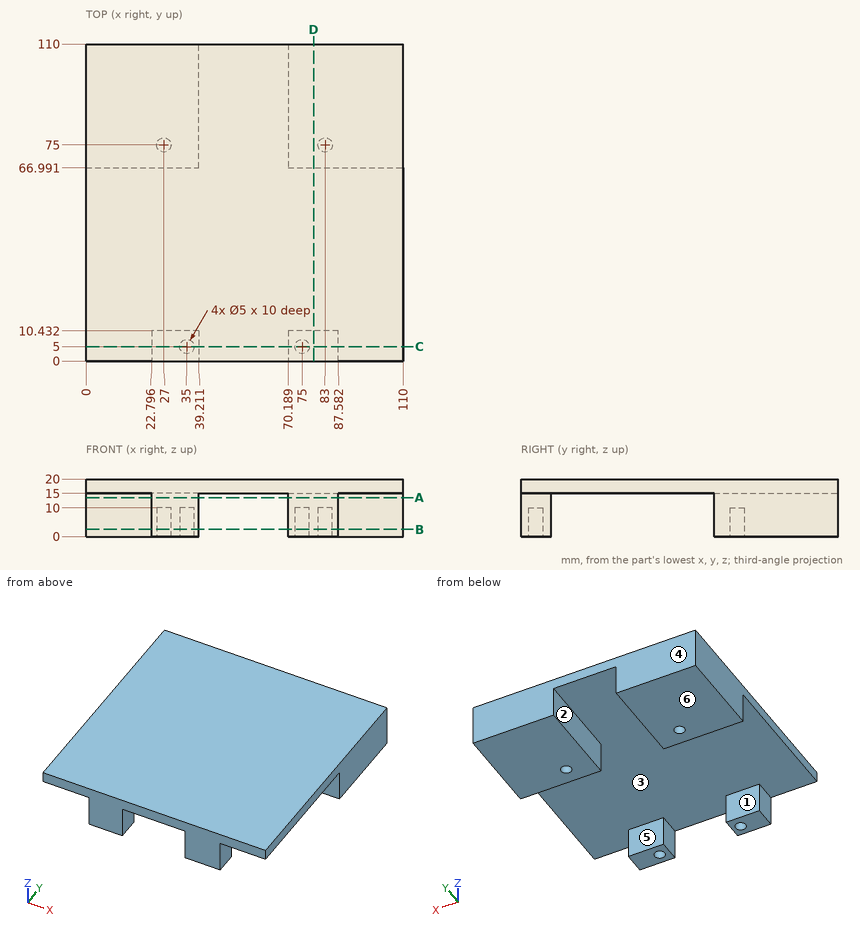
Here's the drawing with two shaded views (mm, measured from the low corner). I have some questions. A direction names the side the tool comes from. Give positions to 0.01 mm unless a question says otherwise; leave off trailing zeros. Write each loop counter-clockwise with the first axis right and the second up, starting at its lowest first coordinate (ties: lowest second). Pieces come first, ordered by that corner, then holes. Notation, with made-up numbers: (33, 14.25) -> (49, 14.25) arc R35 ccw to (49, 51.25) -> close; hole circle Ø10 at (-4, 57.25). An arc over 180 degrees is marked (long way). Answer as a JSON object with one key per item and string values. Group by question number.
Item 1: We'd pull the mould along Y, two halves only. Please class the marked faces 4, 5 and 6: +Y half, -Y half, draft (parallel to the pull), parting line (faces both ways), or undercut.
Item 2: Suppose I cut it at D-D (x = 79). Please give me the cut outline in (y, z), plus the area to 3 significant figures.
Item 3: Please list where these lines run through material, in increasing order: line 1 (X direction, y = 75, z = 3.5); line 2 (X direction, y = 5, z = 2) (1 decimal); line 3 (X direction, y = 72, z = 12.75). Write a range as [from, to].
Item 4: For the marked faces 1, 2 and 3, which set-ups out of +Z, -Z, +X, -X, +Y, -Y let a thin tool reach every point of the face, with its end or its side?
Item 5: I'm going to push flat-ended pins straight in: P1, Ø1.5, axis at x = 82.5, y = 76, coming from the -Z side; P2, Ø8.5, axis at y = 6, z = 8, coming from the -X side; P3, Ø7.5, axis at x = 19, z = 6, coming from the -Y side. Where does each tip first touch, or does it pass through?
Item 6: Suppose I cut it at C-C (y = 5). Please give me the cut outline in (x, z) (1 decimal).
Item 7: Suppose I cut it at B-B (z = 2.5). Please give me the cut outline in (x, y) (1 decimal).
Item 8: Suppose I cut it at A-A (z = 13.5). Please give me the cut outline in (x, y) (1 decimal).
Findings:
{
 "1": {"face 4": "+Y half", "face 5": "undercut", "face 6": "draft"},
 "2": {"outline": "(0, 0) -> (10.43, 0) -> (10.43, 15) -> (66.99, 15) -> (66.99, 0) -> (110, 0) -> (110, 20) -> (0, 20) -> close", "area": "1,350 mm²"},
 "3": {"line 1": "x = [0, 24.5], [29.5, 39.21], [70.19, 80.5], [85.5, 110]", "line 2": "x = [22.8, 32.5], [37.5, 39.2], [70.2, 72.5], [77.5, 87.6]", "line 3": "x = [0, 39.21], [70.19, 110]"},
 "4": {"face 1": "-Z, +X, -X", "face 2": "-Z, +Y, -Y", "face 3": "-Z"},
 "5": {"P1": "stops at z = 10", "P2": "stops at x = 22.8", "P3": "stops at y = 66.99"},
 "6": {"outline": "(0, 15) -> (22.8, 15) -> (22.8, 0) -> (32.5, 0) -> (32.5, 10) -> (37.5, 10) -> (37.5, 0) -> (39.2, 0) -> (39.2, 15) -> (70.2, 15) -> (70.2, 0) -> (72.5, 0) -> (72.5, 10) -> (77.5, 10) -> (77.5, 0) -> (87.6, 0) -> (87.6, 15) -> (110, 15) -> (110, 20) -> (0, 20) -> close"},
 "7": {"outline": "(0, 67) -> (39.2, 67) -> (39.2, 110) -> (0, 110) -> close; (22.8, 0) -> (39.2, 0) -> (39.2, 10.4) -> (22.8, 10.4) -> close; (70.2, 0) -> (87.6, 0) -> (87.6, 10.4) -> (70.2, 10.4) -> close; (70.2, 67) -> (110, 67) -> (110, 110) -> (70.2, 110) -> close; hole circle Ø5 at (27, 75); hole circle Ø5 at (35, 5); hole circle Ø5 at (75, 5); hole circle Ø5 at (83, 75)"},
 "8": {"outline": "(0, 67) -> (39.2, 67) -> (39.2, 110) -> (0, 110) -> close; (22.8, 0) -> (39.2, 0) -> (39.2, 10.4) -> (22.8, 10.4) -> close; (70.2, 0) -> (87.6, 0) -> (87.6, 10.4) -> (70.2, 10.4) -> close; (70.2, 67) -> (110, 67) -> (110, 110) -> (70.2, 110) -> close"}
}
